The listing builds one solid part. Answer for the finished solid, in the listing's coordinates (mm). Give positions to 0.01 mm unless a question says otherwise; leave off trailing zeros. Write each loop counter-clockwise with the first axis right and the second up, starting at its lowest first coordinate (ties: lowest second). Pieces come first, ordered by that corner, then holes. Notation, with made-up numbers: (-22, 50.5) - (-1, 50.5) arc R34 cw to (-1, 81.5) - close; hole circle Ø7 at (33.5, -35). An arc over 180 degrees is marked (long way). Write each question's results on one line, items separated by ' | '. Start each with the question number.
Q1. Find the intervals of material crossed by probe 1 along Y at (x, z) = (9, 18); probe 2 along X at (y, z) = (-5, 13); probe 3 along X at (y, z) = (-19, 26.5), in increasing order.
Q2. Section B-B (y = 20) is taken. Determine the outline of the cut face in (x, z), plus the area to 3 significant figures.
Q3. Section C-C (z = 29.5) is taken. State how many separate pieces and enclosed holes the cut face has, plus the area to 3 significant figures.
Q4. Section A-A (x = 9) is taken. Determine the outline of the cut face in (y, z).
```python
from build123d import *

# Parameters (mm, degrees)
SKETCH_1_R      = 2
EXTRUDE_1_DEPTH = 32


with BuildPart() as part:
    # 草图1 → 凸台-拉伸1 (new body)
    with BuildSketch(Plane.XY):
        with BuildLine():
            Line((12, 28), (-12, 28))
            ThreePointArc((-12, 28), (-14.828427125, 26.828427125), (-16, 24))
            Line((-16, 24), (-16, -24))
            ThreePointArc((-16, -24), (-14.828427125, -26.828427125), (-12, -28))
            Line((-12, -28), (12, -28))
            ThreePointArc((12, -28), (14.828427125, -26.828427125), (16, -24))
            Line((16, -24), (16, 24))
            ThreePointArc((16, 24), (14.828427125, 26.828427125), (12, 28))
        make_face()
        with Locations((9, 20)):
            Circle(SKETCH_1_R, mode=Mode.SUBTRACT)
        with Locations((9, 6.666666667)):
            Circle(SKETCH_1_R, mode=Mode.SUBTRACT)
        with Locations((9, -6.666666667)):
            Circle(SKETCH_1_R, mode=Mode.SUBTRACT)
        with Locations((9, -20)):
            Circle(SKETCH_1_R, mode=Mode.SUBTRACT)
        with Locations(Location((-9, -20, 0), (0, 0, 180))):
            Circle(SKETCH_1_R, mode=Mode.SUBTRACT)
        with Locations(Location((-9, -6.666666667, 0), (0, 0, 180))):
            Circle(SKETCH_1_R, mode=Mode.SUBTRACT)
        with Locations(Location((-9, 6.666666667, 0), (0, 0, 180))):
            Circle(SKETCH_1_R, mode=Mode.SUBTRACT)
        with Locations(Location((-9, 20, 0), (0, 0, 180))):
            Circle(SKETCH_1_R, mode=Mode.SUBTRACT)
    extrude(amount=EXTRUDE_1_DEPTH)


solid = part.part
```
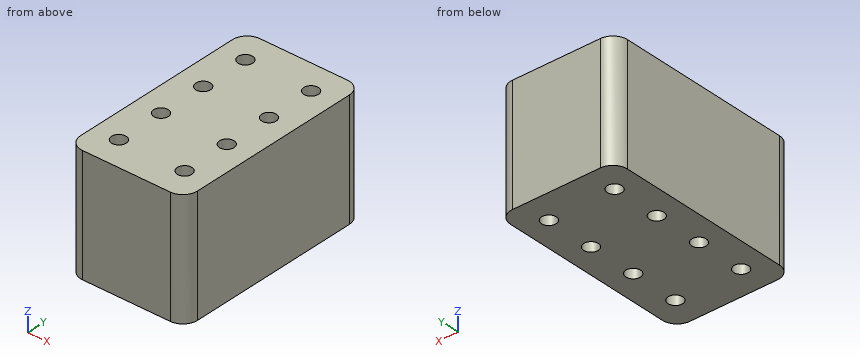
Answers below:
1) probe 1: y = -28 to -22, -18 to -8.67, -4.67 to 4.67, 8.67 to 18, 22 to 28 | probe 2: x = -16 to -10.11, -7.89 to 7.89, 10.11 to 16 | probe 3: x = -16 to -10.73, -7.27 to 7.27, 10.73 to 16
2) outline: (-16, 0) - (-11, 0) - (-11, 32) - (-16, 32) - close; (-7, 0) - (7, 0) - (7, 32) - (-7, 32) - close; (11, 0) - (16, 0) - (16, 32) - (11, 32) - close | area: 768 mm2
3) separate pieces: 1 | enclosed holes: 8 | area: 1,680 mm2
4) outline: (-28, 0) - (-22, 0) - (-22, 32) - (-28, 32) - close; (-18, 0) - (-8.67, 0) - (-8.67, 32) - (-18, 32) - close; (-4.67, 0) - (4.67, 0) - (4.67, 32) - (-4.67, 32) - close; (8.67, 0) - (18, 0) - (18, 32) - (8.67, 32) - close; (22, 0) - (28, 0) - (28, 32) - (22, 32) - close
